Design review of the part built by this model. Coordinates are the model's own, in mm. A direction names the side the tool comes from. Give positions to 0.01 mm unless a question says otherwise; leave off trailing zeros. Loops run counter-clockwise (first coordinate to the right, second up) from the corner with the lowest first, then second, coordinate; pieces in that order, holes last. Notation, with made-up numbers: M -17.5,40 L -13.5,40 A16 ccw -13.5,58 Z; hole C 32,26.5 d9. An arc over 180 degrees is marked long. Answer as CSV lines item,"result".
Autodesk Inventor part; units mm, degrees
ref_plane "YZ Plane" through (0, 0, 0) normal (1, 0, 0) x (0, 1, 0)
ref_plane "XZ Plane" through (0, 0, 0) normal (0, 1, 0) x (-1, 0, 0)
ref_plane "XY Plane" through (0, 0, 0) normal (0, 0, 1) x (1, 0, 0)
sketch "Sketch1" plane through (0, 0, 0) normal (0, 0, 1) x (1, 0, 0)
  line L0 (-34.86, 0) -> (34.86, 0) construction
  line L1 (0, -34.86) -> (0, 34.86) construction
  line L2 (0, 0) -> (11.1575, 11.1575) construction
  line L3 (0, 0) -> (15.7791, 0) construction
  line L4 (0, 24.9) -> (16.8009, 24.9)
  line L5 (16.8009, 24.9) -> (16.8009, 21.2415)
  line L6 (16.8009, 21.2415) -> (19.0212, 19.0212)
  line L7 (24.9, 0) -> (24.9, 16.8009)
  line L8 (24.9, 16.8009) -> (21.2415, 16.8009)
  line L9 (21.2415, 16.8009) -> (19.0212, 19.0212)
  line L10 (0, -24.9) -> (16.8009, -24.9)
  line L11 (16.8009, -24.9) -> (16.8009, -21.2415)
  line L12 (16.8009, -21.2415) -> (19.0212, -19.0212)
  line L13 (24.9, 0) -> (24.9, -16.8009)
  line L14 (24.9, -16.8009) -> (21.2415, -16.8009)
  line L15 (21.2415, -16.8009) -> (19.0212, -19.0212)
  line L16 (0, 24.9) -> (-16.8009, 24.9)
  line L17 (-16.8009, 24.9) -> (-16.8009, 21.2415)
  line L18 (-16.8009, 21.2415) -> (-19.0212, 19.0212)
  line L19 (-24.9, 16.8009) -> (-21.2415, 16.8009)
  line L20 (-21.2415, 16.8009) -> (-19.0212, 19.0212)
  line L21 (0, -24.9) -> (-16.8009, -24.9)
  line L22 (-16.8009, -24.9) -> (-16.8009, -21.2415)
  line L23 (-16.8009, -21.2415) -> (-19.0212, -19.0212)
  line L24 (-21.2415, -16.8009) -> (-19.0212, -19.0212)
  line L25 (-24.9, -16.8009) -> (-21.2415, -16.8009)
  line L26 (-24.9, 0) -> (-24.9, -16.8009)
  line L27 (-24.9, 0) -> (-24.9, 16.8009)
  circle A0 centre (0, 0) radius 12.5
  dimension "d0" = 45
  dimension "d2" = 24.9
  dimension "d3" = 3.14
  dimension "d4" = 26.9
  dimension "d5" = 25
extrude "Extrusion1" add sketch "Sketch1" along normal blind 5
sketch "Sketch2" plane through (0, 0, 5) normal (0, 0, 1) x (1, 0, 0)
  circle A0 centre (0, 0) radius 12.5
  line L0 (16.8009, 24.9) -> (-16.8009, 24.9)
  line L1 (-16.8009, 24.9) -> (-16.8009, 21.2415)
  line L2 (-16.8009, 21.2415) -> (-21.2415, 16.8009)
  line L3 (-21.2415, 16.8009) -> (-24.9, 16.8009)
  line L4 (-24.9, 16.8009) -> (-24.9, -16.8009)
  line L5 (-24.9, -16.8009) -> (-21.2415, -16.8009)
  line L6 (-21.2415, -16.8009) -> (-16.8009, -21.2415)
  line L7 (-16.8009, -21.2415) -> (-16.8009, -24.9)
  line L8 (-16.8009, -24.9) -> (16.8009, -24.9)
  line L9 (16.8009, -24.9) -> (16.8009, -21.2415)
  line L10 (16.8009, -21.2415) -> (21.2415, -16.8009)
  line L11 (21.2415, -16.8009) -> (24.9, -16.8009)
  line L12 (24.9, -16.8009) -> (24.9, 16.8009)
  line L13 (24.9, 16.8009) -> (21.2415, 16.8009)
  line L14 (21.2415, 16.8009) -> (16.8009, 21.2415)
  line L15 (16.8009, 21.2415) -> (16.8009, 24.9)
  line L16 (-34.86, 0) -> (34.86, 0) construction
  line L17 (0, -34.86) -> (0, 34.86) construction
  line L18 (-10, 21.9) -> (10, 21.9)
  line L19 (10, 21.9) -> (10, 18.9)
  line L20 (10, 18.9) -> (-10, 18.9)
  line L21 (-10, 18.9) -> (-10, 21.9)
  line L22 (-10, -21.9) -> (10, -21.9)
  line L23 (10, -21.9) -> (10, -18.9)
  line L24 (10, -18.9) -> (-10, -18.9)
  line L25 (-10, -18.9) -> (-10, -21.9)
  dimension "d8" = 20
  dimension "d9" = 3
  dimension "d10" = 3
extrude "Extrusion2" add sketch "Sketch2" along normal blind 7 contours L18 L19 L20 L21 | L25 L24 L23 L22
chamfer "Fase1" distance 1.5 distance2 7 1 edges at (0, 21.9, 12) measured on face at (-3.3333, 19.9, 12)
chamfer "Fase2" distance 1.5 distance2 7 1 edges at (0, -21.9, 12) measured on face at (-3.3333, -19.9, 12)
properties part number "20_Cube_insert_Sample_holder"
1. We need section C-C, the plane z = 6.25. Write out the cut boundary in (x, y).
Answer block:
outline,"M -10,-21.63 L 10,-21.63 L 10,-18.9 L -10,-18.9 Z; M -10,18.9 L 10,18.9 L 10,21.63 L -10,21.63 Z"
2. For faces 1 (the flat face through (16.801, -23, 2)), 2 (the flat face through (-10, -20, 8)), 3 (the flat face through (0, -18.9, 8)), 4 (the flat face through (-23, 16.801, 2)), list the 3-axis set-ups (+Z, -Z, +X, -X, +Y, -Y) from which the entire face can be reached by the end or side of a thin tool; tool diameter is ignored.
Answer block:
face 1,"+Z, -Z, +X, -Y"
face 2,"+Z, -X, +Y, -Y"
face 3,"+Z, +X, -X"
face 4,"+Z, -Z, -X, +Y"
3. The part is to be moulded in two halves that separate along Y. For faces 5 (the flat face through (23, 16.801, 2)), 6 (the cylindrical face through (11.923, -3.755, 2.465)), 7 (the flat face through (0, 20, 12)), say which applies: pulls with the +Y half, pulls with the -Y half, needs draft (parallel to the pull), parting line crosses it, or undercut.
Answer block:
face 5,"pulls with the +Y half"
face 6,"undercut"
face 7,"needs draft"
4. We need section B-B, the plane y = -3.5. Write out the cut boundary in (x, z).
Answer block:
outline,"M -24.9,0 L -12,0 L -12,5 L -24.9,5 Z; M 12,0 L 24.9,0 L 24.9,5 L 12,5 Z"
5. To check wall thickness, follow L1, parallel to Y at x = 0, z = 3; L2, parallel to X at y = 20.5, z = 10.5; L3, parallel to Z at x = -5.5, y = -16.5. State the ranges of each line that lie inside material, in increasing order. Write a range as [from, to].
Answer block:
L1,"[-24.9, -12.5], [12.5, 24.9]"
L2,"[-10, 10]"
L3,"[0, 5]"
6. For P1, Ø4, axis at y = -24, z = 2.5, coming from the +X side; P2, Ø0.9, axis at y = 21, z = 10, coming from the -X side; P3, Ø5, axis at x = 11, y = -1.5, coming from the +Z side; P4, Ø3, axis at x = -13, z = 7, coming from the +Y side, all flat-tipped, find the tip position at first contact; note any pin that passes through.
Answer block:
P1,"x = 16.8"
P2,"x = -10"
P3,"z = 5"
P4,"through"
